The listing builds one solid part. Answer for the finished solid, in the listing's coordinates (mm). A direction names the side the tool comes from. Give positions to 0.01 mm unless a question says otherwise; leave off trailing zeros. Loops run counter-clockwise (first coordinate to the right, second up) from the corner with the lowest first, then second, coordinate; pieces in that order, holes last. Notation, with made-up numbers: (34.25, 0) - (48.25, 0) arc R17 ccw to (48.25, 16) - close; hole circle Ø2 at (23.5, -11). An arc over 180 degrees is marked (long way). Write item = value, one per line. Start each with the question number.
1) Flat-ended cylindrical pins translate along their axes: P1, Ø4.5, axis at x = -140, z = 0, coming from the -Y side (3 decimals); P2, Ø6, axis at x = -35, z = 0, coming from the +Y side; P3, Ø6, axis at x = -55, z = 0, coming from the +Y side. Find the tip coordinate at first contact, or state that the pin passes through.
2) Consider probe 1 along Z at (x, y) = (-140, 1); probe 2 along Y at (x, z) = (-17, 20); probe 3 along X at (y, z) = (34, -6.5). Determine where each line is inside the solid, lowest interval first.
3) The part is cut by section C-C on x = 0. Write down the section's boundary in (y, z), plus the area to 3 significant figures.
4) The part is cut by section B-B on y = 61.5. Write down the section's boundary in (x, z), plus the area to 3 significant figures.
5) Which of the six approach directions +Z, -Z, +X, -X, +Y, -Y give full straight-line access (tool end or side, diameter ignored) to faces 1 (the flat face through (-15, 176, -3)), 2 (the flat face through (-125, 5, -2)), 3 (the flat face through (-22, 5, 18)), 4 (the flat face through (-126.17, 91.63, -2.33))?
6) The part is cut by section A-A on x = -148. Write down the section's boundary in (y, z), plus the area to 3 significant figures.
7) The mould has two halves that part along Y. Classify faces 5 (the flat face through (-125, 10, 5)), 6 (the flat face through (-24, -5, 30)), 7 (the flat face through (-138.25, 88.655, -2.535)), 8 (the flat face through (-14, -20, 3)): +Y half, -Y half, draft (parallel to the pull), parting line (faces both ways), or undercut.
from build123d import *

# Parameters (mm, degrees)
PAD_DEPTH            = 20
PAD_DEPTH_BACK       = 180
PAD001_DEPTH         = 25
POCKET_DEPTH         = 180.001
POCKET_DEPTH_BACK    = 20.001
PAD002_DEPTH         = 20
PAD002_DEPTH_BACK    = 5
SKETCH008_W          = 20.2
SKETCH008_H          = 20.2
POCKET001_DEPTH      = 15.001
POCKET001_DEPTH_BACK = 30.001
SKETCH009_R          = 2.6
POCKET002_DEPTH      = 5
SKETCH010_R          = 5
POCKET003_DEPTH      = 10
SKETCH011_R          = 2.6
POCKET004_DEPTH      = 265.001
SKETCH012_R          = 5
POCKET005_DEPTH      = 20
SKETCH013_R          = 2
POCKET006_DEPTH      = 180.001


with BuildPart() as part:
    # Sketch → Pad (new body, two sides)
    with BuildSketch(Plane.XZ) as pad_sk:
        with BuildLine():
            Line((-15, 10), (3.201562, 10))
            Line((3.201562, 10), (6.201562, 10))
            ThreePointArc((15, -3.65795), (12.609975, 4.465345), (6.201562, 10))
            Line((15, -3.65795), (15, -15))
            Line((15, -15), (-15, -15))
            Line((-15, -15), (-15, 10))
        make_face()
    extrude(amount=PAD_DEPTH)
    extrude(pad_sk.sketch, amount=-PAD_DEPTH_BACK)

    # AdditivePipe: sweep along a path in Sketch001
    with BuildLine(Plane.XY) as additivepipe_path:
        Line((-265, 0), (0, 0))
    # Sketch002 (on DatumPlane) → AdditivePipe (sweep)
    with BuildSketch(Plane.YZ.offset(-265)):
        Polygon((0, -10), (0, 10), (15, 10), (5, 0), (5, -5), (15, -15), (-5, -15), (-5, -10), align=None)
    sweep(path=additivepipe_path.line, is_frenet=True)

    # AdditivePipe001: sweep along a path in Sketch004
    with BuildLine(Plane.XY) as additivepipe001_path:
        Line((-265, 0), (-15, 165))
    # Sketch003 (on DatumPlane) → AdditivePipe001 (sweep)
    with BuildSketch(Plane.YZ.offset(-265)):
        Polygon((0, 10), (0, -15), (15, -15), (5, -5), (5, 0), (15, 10), align=None)
    sweep(path=additivepipe001_path.line, is_frenet=True)

    # Sketch005 (on Face19 of AdditivePipe001) → Pad001 (join)
    with BuildSketch(Plane(origin=(0, 0, 10), x_dir=(-1, 0, 0), z_dir=(0, 0, 1))):
        with BuildLine():
            ThreePointArc((238.103146, -17.751924), (238.71354, -16.068657), (237.276897, -15))
            Line((237.276897, -15), (237.276897, -5))
            Line((237.276897, -5), (257.424242, -5))
            Line((257.424242, -5), (257.424242, -10))
            Line((257.424242, -10), (241.155013, -20.737691))
            Line((241.155013, -20.737691), (238.103146, -17.751924))
        make_face()
        with BuildLine():
            ThreePointArc((15, -162.212752), (15.789148, -163.533619), (17.326253, -163.464673))
            Line((17.326253, -163.464673), (19.815663, -166.821662))
            Line((19.815663, -166.821662), (12.527544, -171.631821))
            Line((12.527544, -162.212752), (12.527544, -171.631821))
            Line((15, -162.212752), (12.527544, -162.212752))
        make_face()
    extrude(amount=-PAD001_DEPTH)

    # Sketch006 → Pocket (cut, two sides)
    with BuildSketch(Plane.XZ) as pocket_sk:
        with BuildLine():
            ThreePointArc((-8, 6.954135), (0, -10.6), (8, 6.954135))
            Line((8, 22.954135), (8, 6.954135))
            Line((-8, 22.954135), (8, 22.954135))
            Line((-8, 6.954135), (-8, 22.954135))
        make_face()
    extrude(amount=-POCKET_DEPTH, mode=Mode.SUBTRACT)
    extrude(pocket_sk.sketch, amount=POCKET_DEPTH_BACK, mode=Mode.SUBTRACT)

    # Sketch007 → Pad002 (join, two sides)
    with BuildSketch(Plane.XZ) as pad002_sk:
        Polygon((-8, 10), (-20, 30), (-30, 30), (-30, -15), (-10.6, -15), (-10.6, 6.954135), (-8, 6.954135), align=None)
    extrude(amount=PAD002_DEPTH)
    extrude(pad002_sk.sketch, amount=-PAD002_DEPTH_BACK)

    # Sketch008 → Pocket001 (cut, two sides)
    with BuildSketch(Plane.XY) as pocket001_sk:
        with Locations((-35.1, -10.1)):
            Rectangle(SKETCH008_W, SKETCH008_H)
    extrude(amount=-POCKET001_DEPTH, mode=Mode.SUBTRACT)
    extrude(pocket001_sk.sketch, amount=POCKET001_DEPTH_BACK, mode=Mode.SUBTRACT)

    # Sketch009 → Pocket002 (cut)
    with BuildSketch(Plane.XZ):
        with Locations((-35, 0)):
            Circle(SKETCH009_R)
        with Locations((-55, 0)):
            Circle(SKETCH009_R)
        with Locations((-140, 0)):
            Circle(SKETCH009_R)
        with Locations((-225, 0)):
            Circle(SKETCH009_R)
    extrude(amount=-POCKET002_DEPTH, mode=Mode.SUBTRACT)

    # Sketch010 (on DatumPlane) → Pocket003 (cut)
    with BuildSketch(Plane.XZ.offset(-15)):
        with Locations((-225, 0)):
            Circle(SKETCH010_R)
        with Locations((-140, 0)):
            Circle(SKETCH010_R)
        with Locations((-55, 0)):
            Circle(SKETCH010_R)
        with Locations((-35, 0)):
            Circle(SKETCH010_R)
    extrude(amount=POCKET003_DEPTH, mode=Mode.SUBTRACT)

    # Sketch011 → Pocket004 (cut, through all)
    with BuildSketch(Plane.YZ):
        with Locations((-10, 20)):
            Circle(SKETCH011_R)
    extrude(amount=-POCKET004_DEPTH, mode=Mode.SUBTRACT)

    # Sketch012 → Pocket005 (cut)
    with BuildSketch(Plane.YZ):
        with Locations((-10, 20)):
            Circle(SKETCH012_R)
    extrude(amount=-POCKET005_DEPTH, mode=Mode.SUBTRACT)

    # Sketch013 → Pocket006 (cut, through all)
    with BuildSketch(Plane.XZ):
        with Locations((-225, 0)):
            Circle(SKETCH013_R)
    extrude(amount=-POCKET006_DEPTH, mode=Mode.SUBTRACT)


solid = part.part
Answer below:
q1.P1 = 81.015
q1.P2 = 160.39
q1.P3 = 147.19
q2.probe_1 = -15 to -2.6, 2.6 to 10
q2.probe_2 = -20 to -15, -5 to 5
q2.probe_3 = -223.33 to -213.48, -15 to -8.37, 8.37 to 15
q3.outline = (-20, -15) - (180, -15) - (180, -10.6) - (-20, -10.6) - close
q3.area = 880 mm2
q4.outline = (-194.55, -15) - (-171.82, -15) - (-171.82, 10) - (-194.55, 10) - (-179.39, 0) - (-179.39, -5) - close; (-15, -15) - (15, -15) - (15, -3.66) arc R15 ccw to (8, 9.03) - (8, 6.95) arc R10.6 cw (long way) to (-8, 6.95) - (-8, 10) - (-15, 10) - close
q4.area = 697 mm2
q5.face_1 = -X, +Y
q5.face_2 = none
q5.face_3 = +Z, +X, -X, +Y
q5.face_4 = +Z, -Z
q6.outline = (-5, -15) - (15, -15) - (5, -5) - (5, 0) - (15, 10) - (0, 10) - (0, -10) - (-5, -10) - close; (77.22, -15) - (92.22, -15) - (82.22, -5) - (82.22, 0) - (92.22, 10) - (77.22, 10) - close
q6.area = 475 mm2
q7.face_5 = undercut
q7.face_6 = draft
q7.face_7 = +Y half
q7.face_8 = -Y half
